```python
from build123d import *

# Parameters (mm, degrees)
F0_W     = 169
F0_H     = 75
F0_R     = 6
F1_DEPTH = 1.75
F2_W     = 164
F2_H     = 75
F3_DEPTH = 1.5
F4_R     = 5
F5_DEPTH = 25


with BuildPart() as f1:
    # F0 (on Top) → F1 (new body)
    with BuildSketch(Plane.XY):
        Rectangle(F0_W, F0_H)
        with Locations((-42.25, 0)):
            Circle(F0_R, mode=Mode.SUBTRACT)
        with Locations((42.25, 0)):
            Circle(F0_R, mode=Mode.SUBTRACT)
    extrude(amount=F1_DEPTH)

    # F2 (on face) → F3 (join)
    with BuildSketch(Plane.XY.offset(1.75)):
        Rectangle(F2_W, F2_H)
    extrude(amount=F3_DEPTH)

    # F4
    f4_edges = [f1.edges().sort_by_distance(p)[0] for p in [
        (-84.5, -37.5, 0.875),
        (84.5, -37.5, 0.875),
        (84.5, 37.5, 0.875),
        (-84.5, 37.5, 0.875),
    ]]
    fillet(f4_edges, radius=F4_R)

    # F0 (on Top) → F5 (cut)
    with BuildSketch(Plane.XY):
        with Locations((42.25, 0)):
            Circle(F0_R)
        with Locations((-42.25, 0)):
            Circle(F0_R)
    extrude(amount=F5_DEPTH, mode=Mode.SUBTRACT)


solid = f1.part
```
The model under review builds one solid part; all positions refer to its coordinate system, in mm. Round coordinates to 2 decimals unless told otherwise and drop trailing zeros. Write each loop counter-clockwise with the first axis right and the second up, starting at its lowest first coordinate (ties: lowest second). Pieces come first, ordered by that corner, then holes. Notation, with made-up numbers: (11, 0) - (38, 0) arc R28 ccw to (38, 24) - close; hole circle Ø2 at (-24.5, -8). An arc over 180 degrees is marked (long way). Use one line per item in the form item = value.
Q1. Draft analysis for pull direction Y (two halves, no side actions). For faces 1 (the cylindrical face through (-82.32, -36.63, 1.29)), 2 (the cylindrical face through (36.256, 0.264, 1.602)), 3 (the flat face through (-1, 37.5, 2)), 4 (the flat face through (-1, 1, 0)), state which applies: +Y half, -Y half, draft (parallel to the pull), parting line (faces both ways), or undercut.
Answer key:
face_1 = -Y half
face_2 = undercut
face_3 = +Y half
face_4 = draft
Q2. Consider section C-C (y = 0). State the section outline as (x, z) points, and give its area (3 significant figures).
Answer key:
outline = (-84.5, 0) - (-48.25, 0) - (-48.25, 3.25) - (-82, 3.25) - (-82, 1.75) - (-84.5, 1.75) - close; (-36.25, 0) - (36.25, 0) - (36.25, 3.25) - (-36.25, 3.25) - close; (48.25, 0) - (84.5, 0) - (84.5, 1.75) - (82, 1.75) - (82, 3.25) - (48.25, 3.25) - close
area = 464 mm2
Q3. For line 1 (X direction, y = 0, z = 2.55); line 2 (Y direction, x = 42.25, z = 1.65); line 3 (X direction, y = 0, z = 1.6), list the stretches that pass through material, from the lowest coordinate up. Write a range as [from, to].
Answer key:
line_1 = [-82, -48.25], [-36.25, 36.25], [48.25, 82]
line_2 = [-37.5, -6], [6, 37.5]
line_3 = [-84.5, -48.25], [-36.25, 36.25], [48.25, 84.5]
Q4. Consider section A-A (x = 42.25). State the section outline as (y, z) points, and give its area (3 significant figures).
Answer key:
outline = (-37.5, 0) - (-6, 0) - (-6, 3.25) - (-37.5, 3.25) - close; (6, 0) - (37.5, 0) - (37.5, 3.25) - (6, 3.25) - close
area = 205 mm2
Q5. Insertion check: pin 1 Ø3 at (x, y) = (-83, -5) entering from +Z; pin 2 Ø0.8 at (y, z) = (-4, 2.5) entering from +X; pin 3 Ø0.8 at (x, y) = (83, 12) entering from +Z. Each pin has a flat end and moves straight along its axis. Give the tip position at first contact, or say it passes through.
Answer key:
pin_1 = 3.25
pin_2 = 82
pin_3 = 1.75
Q6. Consider section B-B (z = 1). State the section outline as (x, y) points.
Answer key:
outline = (-84.5, -32.5) arc R5 ccw to (-79.5, -37.5) - (79.5, -37.5) arc R5 ccw to (84.5, -32.5) - (84.5, 32.5) arc R5 ccw to (79.5, 37.5) - (-79.5, 37.5) arc R5 ccw to (-84.5, 32.5) - close; hole circle Ø12 at (-42.25, 0); hole circle Ø12 at (42.25, 0)
